Geometry check sheet. Reference: the model listing, model coordinates, mm. A direction names the side the tool comes from. Give positions to 0.01 mm unless a question says otherwise; leave off trailing zeros. Write each loop counter-clockwise with the first axis right and the second up, starting at its lowest first coordinate (ties: lowest second). Pieces come first, ordered by that corner, then holes. Notation, with made-up numbers: (14.5, -37) -> (66.5, -37) arc R10 cw to (66.5, -29) -> close; hole circle Ø3 at (7, -9). An arc over 180 degrees is marked (long way). One line per item, written item: value.
from build123d import *

# Parameters (mm, degrees)
F1_DEPTH = 25
F2_W     = 34.969408
F2_H     = 15.419583
F3_DEPTH = 25


with BuildPart() as f1:
    # F0 (on Front) → F1 (new body)
    with BuildSketch(Plane.XZ):
        Polygon((15.279747, 22.047983), (0, 22.047983), (-15.279747, 22.047983), (-15.279747, 32.078233), (-52.158151, 32.078233), (-57.22541, 27.396761), (-57.22541, 12.758005), (-57.22541, -22.994338), (-52.158151, -29.46917), (-15.279747, -29.46917), (-15.279747, -20.179192), (0, -20.179192), (15.279747, -20.179192), (15.279747, -29.46917), (52.158151, -29.46917), (57.22541, -22.994338), (57.22541, 12.758005), (57.22541, 27.396761), (52.158151, 32.078233), (15.279747, 32.078233), align=None)
    extrude(amount=F1_DEPTH)

    # F2 (on face) → F3 (cut)
    with BuildSketch(Plane.XZ.offset(25)):
        with Locations((0, 0.137676)):
            Rectangle(F2_W, F2_H)
    extrude(amount=-F3_DEPTH, mode=Mode.SUBTRACT)


solid = f1.part
1) Sectioned sample at B-B on y = -21.75. Record the cut outline in (x, z), plus the area to 3 significant figures.
Verdict:
outline: (-57.23, -22.99) -> (-52.16, -29.47) -> (-15.28, -29.47) -> (-15.28, -20.18) -> (15.28, -20.18) -> (15.28, -29.47) -> (52.16, -29.47) -> (57.23, -22.99) -> (57.23, 27.4) -> (52.16, 32.08) -> (15.28, 32.08) -> (15.28, 22.05) -> (-15.28, 22.05) -> (-15.28, 32.08) -> (-52.16, 32.08) -> (-57.23, 27.4) -> close; hole (-17.48, -7.57) -> (17.48, -7.57) -> (17.48, 7.85) -> (-17.48, 7.85) -> close
area: 5,860 mm^2
2) Sectioned sample at A-A on x = 10. Record the cut outline in (y, z), plus the area to 3 significant figures.
Verdict:
outline: (-25, -20.18) -> (0, -20.18) -> (0, -7.57) -> (-25, -7.57) -> close; (-25, 7.85) -> (0, 7.85) -> (0, 22.05) -> (-25, 22.05) -> close
area: 670 mm^2
3) Tool access check on faces 1 (the flat face through (-17.485, -13, 0)), 2 (the flat face through (-1, 0, 9)), 3 (the flat face through (0, -12, 22.048)), 4 (the flat face through (33, -12, -29.469)), 5 (the flat face through (-15.28, -12, -25)). Record the directions out of +Z, -Z, +X, -X, +Y, -Y that give a thin tool (end or side, any length) a straight path to the whole face; none if there is none.
Verdict:
face 1: +Y, -Y
face 2: +Z, -Z, +X, -X, +Y
face 3: +Z, +Y, -Y
face 4: -Z, +X, -X, +Y, -Y
face 5: -Z, +Y, -Y
4) Depth check by flat-ended pin: pin 1 Ø4 at (x, y) = (3.5, -15.5) entering from -Z; pin 2 Ø3 at (y, z) = (-10, -26) entering from -X; pin 3 Ø12.5 at (x, y) = (8, -6.5) entering from +Z. Enter the tip coordinate at first touch or a pass-through.
Verdict:
pin 1: z = -20.18
pin 2: x = -56.05
pin 3: z = 22.05
5) Sectioned sample at C-C on z = -4. Record the cut outline in (x, y), plus the area to 3 significant figures.
Verdict:
outline: (-57.23, -25) -> (-17.48, -25) -> (-17.48, 0) -> (-57.23, 0) -> close; (17.48, -25) -> (57.23, -25) -> (57.23, 0) -> (17.48, 0) -> close
area: 1,990 mm^2
6) Scan lines: probe 1 along Z at (x, y) = (6.5, -2.5); probe 2 along X at (y, z) = (-21, -7); probe 3 along X at (y, z) = (-13.75, 25). Record each from-to range of solid material in increasing order.
Verdict:
probe 1: -20.18 to -7.57, 7.85 to 22.05
probe 2: -57.23 to -17.48, 17.48 to 57.23
probe 3: -57.23 to -15.28, 15.28 to 57.23
7) Mould release check, pull along X, two halves, no side actions. Record for faces 6 (the flat face through (-1, -25, 9)), 7 (the flat face through (-54.656, -12.325, 29.77)), 8 (the flat face through (15.28, -12, -25)): released by +X, released by -X, zero draft, split by the parting line, or undercut.
Verdict:
face 6: zero draft
face 7: released by -X
face 8: undercut
